Design review of the part built by this model. Coordinates are the model's own, in mm. Give positions to 0.01 mm unless a question says otherwise; leave off trailing zeros. Order: outer loops, then holes, each group sorted by start corner. A loop starts at its lowest first (then second) coordinate and runs counter-clockwise, first axis right, second up. Notation, with made-up numbers: (82.5, 33) -> (132.5, 33) arc R8 cw to (132.5, 43) -> close; hole circle Ø7 at (35.5, 58). An arc over 180 degrees is marked (long way). Use a Markdown table: item, result. Add a question column.
Autodesk Inventor part; units mm, degrees
ref_plane "YZ Plane" through (0, 0, 0) normal (1, 0, 0) x (0, 1, 0)
ref_plane "XZ Plane" through (0, 0, 0) normal (0, 1, 0) x (-1, 0, 0)
ref_plane "XY Plane" through (0, 0, 0) normal (0, 0, 1) x (1, 0, 0)
sketch "Sketch1" plane through (0, 0, 0) normal (0, 0, 1) x (1, 0, 0)
  line L0 (0, 0) -> (1.6, 0)
  line L1 (1.6, 0) -> (1.6, 700)
  line L2 (1.6, 700) -> (0, 700)
  line L3 (0, 700) -> (0, 0)
  dimension "d0" = 700
  dimension "d1" = 1.6
extrude "Extrusion1" add sketch "Sketch1" along normal blind 1100
sketch "Sketch2" plane through (1.6, 0, 0) normal (0, -1, 0) x (1, 0, 0)
  line L0 (-1.6, 0) -> (-1.6, 1100)
  line L1 (-1.6, 0) -> (0, 0)
  line L2 (-1.6, 0) -> (0, 0)
  line L3 (0, 0) -> (0, 1100)
  line L4 (-1.6, 1100) -> (0, 1100)
  line L5 (-1.6, 0) -> (-1.6, 1100)
extrude "Extrusion2" add sketch "Sketch2" along normal blind 50
sketch "Sketch3" plane through (1.6, 700, 1100) normal (1, 0, 0) x (0, 0, -1)
  line L0 (1100, 0) -> (1100, -750)
  line L1 (1100, -427.9985) -> (1362.866, -427.9985) construction
  line L2 (0, -750) -> (1100, -750)
  circle A0 centre (837.134, -365.688) radius 65
  point P0 (1100, -700)
extrude "Extrusion3" cut sketch "Sketch3" against normal through all
properties part number "cover 2"
1) Add section C-C (x = 0.95). Give the boundary of the cut face in (y, z).
2) Add section B-B (z = 238). Give the boundary of the cut face in (x, y), then the cut area to 3 significant figures.
3) Add section A-A (y = 357). Give the boundary of the cut face in (x, z), then the cut area to 3 significant figures.
4) For L1, parallel to Z at x = 0.55, y = 340; L2, parallel to Z at x = 1.45, y = 293, list the stretches that pass through material, from the lowest coordinate up. Write a range as [from, to].
5) The part is to be moulded in two halves that separate along Z. For faces 1 (the flat face through (1.6, 320, 542)), 2 (the cylindrical face through (0.81, 309.42, 202.82)), say which applies: +Z half, -Z half, draft (parallel to the pull), parting line (faces both ways), or undercut.
Worked answers:
| question | item | result |
|---|---|---|
| 1 | outline | (-50, 0) -> (700, 0) -> (700, 1100) -> (-50, 1100) -> close; hole circle Ø130 at (334.31, 262.87) |
| 2 | outline | (0, -50) -> (1.6, -50) -> (1.6, 274.26) -> (0, 274.26) -> close; (0, 394.37) -> (1.6, 394.37) -> (1.6, 700) -> (0, 700) -> close |
| 2 | area | 1,010 mm^2 |
| 3 | outline | (0, 0) -> (1.6, 0) -> (1.6, 201.95) -> (0, 201.95) -> close; (0, 323.78) -> (1.6, 323.78) -> (1.6, 1100) -> (0, 1100) -> close |
| 3 | area | 1,570 mm^2 |
| 4 | L1 | [0, 198.12], [327.62, 1100] |
| 4 | L2 | [0, 212.68], [313.05, 1100] |
| 5 | face 1 | draft |
| 5 | face 2 | undercut |
